Autodesk Inventor part; units mm, degrees
ref_plane "YZ Plane" through (0, 0, 0) normal (1, 0, 0) x (0, 1, 0)
ref_plane "XZ Plane" through (0, 0, 0) normal (0, 1, 0) x (-1, 0, 0)
ref_plane "XY Plane" through (0, 0, 0) normal (0, 0, 1) x (1, 0, 0)
sketch "Skizze2" plane through (0, 0, 0) normal (0, 0, 1) x (1, 0, 0)
  line L0 (-122.5, 30) -> (122.5, 30)
  line L1 (122.5, 30) -> (122.5, -30)
  line L2 (122.5, -30) -> (-122.5, -30)
  line L3 (-122.5, -30) -> (-122.5, 30)
  line L4 (-122.5, 30) -> (122.5, -30) construction
  line L5 (122.5, 30) -> (-122.5, -30) construction
  point P0 (0, 0)
  dimension "d0" = 245
  dimension "d1" = 60
extrude "Extrusion1" add sketch "Skizze2" along normal blind 2.5
sketch "Skizze3" plane through (0, 0, 2.5) normal (0, 0, 1) x (1, 0, 0)
  line L0 (122.5, 30) -> (-122.5, 30) construction
  line L1 (-122.5, 30) -> (-122.5, -30) construction
  line L2 (-122.5, -30) -> (122.5, -30) construction
  line L3 (122.5, -30) -> (122.5, 30) construction
  line L4 (122.5, 30) -> (-122.5, 30)
  line L5 (122.5, -30) -> (122.5, 30)
  line L6 (-122.5, 30) -> (122.5, 30)
  line L7 (122.5, 30) -> (122.5, 27.5)
  line L8 (122.5, 27.5) -> (-122.5, 27.5)
  line L9 (-122.5, 27.5) -> (-122.5, 30)
  point P0 (0, 0)
  dimension "d4" = 2.5
extrude "Extrusion2" add sketch "Skizze3" along normal blind 20
sketch "Skizze4" plane through (-122.5, 30, 0) normal (0, 1, 0) x (1, 0, 0)
  line L0 (0, 0) -> (245, 0) construction
  line L1 (0, 0) -> (0, -22.5) construction
  line L2 (245, -22.5) -> (0, -22.5) construction
  line L3 (245, 0) -> (245, -22.5) construction
  line L4 (122.5, 0) -> (7, 0) construction
  line L5 (0, 0) -> (245, 0) construction
  line L6 (7, 0) -> (238, 0) construction
  line L7 (7, -22.5) -> (7, -14.5) construction
  line L8 (245, -22.5) -> (0, -22.5)
  line L9 (238, -22.5) -> (238, -14.5) construction
  line L10 (7, -19.5) -> (7, -9.5) construction
  line L11 (9, -19.5) -> (9, -9.5)
  line L12 (5, -9.5) -> (5, -19.5)
  arc A0 (5, -19.5) -> (9, -19.5) centre (7, -19.5) ccw
  arc A1 (9, -9.5) -> (5, -9.5) centre (7, -9.5) ccw
  line L13 (238, -9.5) -> (238, -19.5) construction
  line L14 (236, -9.5) -> (236, -19.5)
  line L15 (240, -19.5) -> (240, -9.5)
  arc A2 (240, -9.5) -> (236, -9.5) centre (238, -9.5) ccw
  arc A3 (236, -19.5) -> (240, -19.5) centre (238, -19.5) ccw
  dimension "d8" = 231
  dimension "d9" = 8
  dimension "d10" = 5
  dimension "d11" = 4
  dimension "d12" = 8
  dimension "d13" = 5
  dimension "d14" = 4
extrude "Extrusion3" cut sketch "Skizze4" against normal blind 20
sketch "Skizze5" plane through (0, 0, 2.5) normal (0, 0, 1) x (1, 0, 0)
  line L0 (122.5, 27.5) -> (-122.5, 27.5) construction
  line L1 (-122.5, 27.5) -> (-122.5, -30) construction
  line L2 (-122.5, -30) -> (122.5, -30) construction
  line L3 (122.5, -30) -> (122.5, 27.5) construction
  line L4 (122.5, -30) -> (122.5, 27.5)
  line L5 (122.5, 27.5) -> (122.5, -30)
  line L6 (122.5, -30) -> (-122.5, -30)
  line L7 (-122.5, -30) -> (-122.5, 27.5)
  line L8 (-122.5, 24.8143) -> (-120.5, 24.8143) construction
  line L9 (122.5, 16.3856) -> (120.5, 16.3856) construction
  line L10 (-122.5, -30) -> (122.5, -30)
  line L11 (0, -30) -> (0, -28) construction
  line L12 (120.5, 27.5) -> (120.5, -28)
  line L13 (120.5, -28) -> (-120.5, -28)
  line L14 (-120.5, -28) -> (-120.5, 27.5)
  line L15 (-122.5, 27.5) -> (-120.5, 27.5)
  line L16 (120.5, 27.5) -> (122.5, 27.5)
  point P0 (0, 0)
  dimension "d17" = 2
  dimension "d18" = 2
  dimension "d19" = 2
extrude "Extrusion4" add sketch "Skizze5" along normal blind 8
fillet "Rundung1" radius 2 7 edges at (-122.5, 30, 11.25) (0, 30, 0) (122.5, 30, 11.25) (0, 30, 22.5) (122.5, 0, 0) (-122.5, 0, 0) (0, -30, 0)
sketch "Skizze7" plane through (0, 0, 0) normal (0, 0, -1) x (-1, 0, 0)
  line L0 (120.5, 30) -> (-120.5, 30) construction
  line L1 (122.5, -30) -> (122.5, 28) construction
  line L2 (-122.5, -30) -> (122.5, -30) construction
  line L3 (-122.5, 28) -> (-122.5, -30) construction
  line L4 (0, 30) -> (0, 0) construction
  line L5 (-102.5, 0.65) -> (102.5, 0.65)
  line L6 (102.5, 0.65) -> (102.5, -0.65)
  line L7 (102.5, -0.65) -> (-102.5, -0.65)
  line L8 (-102.5, -0.65) -> (-102.5, 0.65)
  line L9 (-102.5, 0.65) -> (102.5, -0.65) construction
  line L10 (102.5, 0.65) -> (-102.5, -0.65) construction
  dimension "d28" = 205
  dimension "d29" = 1.3
extrude "Extrusion6" cut sketch "Skizze7" against normal blind 5
sketch "Skizze8" plane through (0, 0, 2.5) normal (0, 0, 1) x (1, 0, 0)
  line L0 (102.5, -0.65) -> (-102.5, -0.65) construction
  line L1 (-102.5, -0.65) -> (102.5, -0.65)
  line L2 (102.5, -0.65) -> (102.5, -2.6532)
  line L3 (102.5, -2.6532) -> (-102.5, -2.6532)
  line L4 (-102.5, -2.6532) -> (-102.5, -0.65)
  point P0 (0, 0)
extrude "Extrusion7" add sketch "Skizze8" along normal blind 5
fillet "Rundung2" radius 2 2 edges at (-102.5, -1.6516, 7.5) (102.5, -1.6516, 7.5)
sketch "Skizze9" plane through (0, 0, 2.5) normal (0, 0, 1) x (1, 0, 0)
  line L0 (-102.5, 0.65) -> (102.5, 0.65) construction
  line L1 (100.5, -0.65) -> (-100.5, -0.65) construction
  line L2 (-102.5, 0.65) -> (102.5, 0.65)
  line L3 (102.5, 0.65) -> (102.5, 1.65)
  line L4 (102.5, 1.65) -> (-102.5, 1.65)
  line L5 (-102.5, 1.65) -> (-102.5, 0.65)
  point P0 (0, 0)
  dimension "d35" = 1
extrude "Extrusion8" cut sketch "Skizze9" against normal blind 10
sketch "Skizze10" plane through (0, 0, 2.5) normal (0, 0, 1) x (1, 0, 0)
  line L0 (-102.5, 1.65) -> (102.5, 1.65)
  line L1 (-102.5, 1.65) -> (102.5, 1.65)
  line L2 (102.5, 1.65) -> (102.5, 3.65)
  line L3 (102.5, 3.65) -> (-102.5, 3.65)
  line L4 (-102.5, 3.65) -> (-102.5, 1.65)
  point P0 (0, 0)
  dimension "d38" = 2
extrude "Extrusion9" add sketch "Skizze10" along normal blind 5
properties part number "Basket" material "Acetalharz, Schwarz"
Geometry: final body of the model. Coordinates: model frame, mm. A direction names the side the tool comes from. Coordinates: 2 decimals unless noted, no trailing zeros. Loops run counter-clockwise (first coordinate to the right, second up) from the corner with the lowest first, then second, coordinate; pieces in that order, holes last. Notation, with made-up numbers: (75, 7) -> (92, 7) arc R20 ccw to (92, 30) -> close; hole circle Ø8 at (-14, -2). An arc over 180 degrees is marked (long way). Use a Markdown table: item, result. Add a question column.
(1) Section query C-C, the plane y = 22. Return loops of the section in (x, z), plus the area to 3 significant figures.
(2) Access query for faces 1 (the flat face through (-1, -0.65, 4)), 2 (the flat face through (2, -28, 6)), 3 (the flat face through (2, -30, 6)). Directions: +Z, -Z, +X, -X, +Y, -Y. A direction counts if a zero-diameter tool reaches every point of the face in a straight line with its end or side. Return the directions, or none.
(3) Section query B-B, the plane x = -22.5. Return loops of the section in (y, z), plus the area to 3 significant figures.
(4) Pin query (flat end, axial travel): pin 1 Ø0.7 at (y, z) = (1, 1) entering from +X; pin 2 Ø1.2 at (y, z) = (29.5, 16) entering from +X; pin 3 Ø2 at (x, y) = (40, 3) entering from +Z. Return the tip coordinate at first contact, or that it passes through.
(5) Line query: line 1 along Y through (x, z) = (37.5, 5.75); line 2 along X through (y, z) = (16.5, 8.25); line 3 along Y through (x, z) = (-43, 8). Output: solid intervals per line, ascending.
(6) Section query A-A, the plane z = 13.5. Return loops of the section in (x, y).
(7) Mould query, pull axis X, two halves, no side actions, for faces 4 (the flat face through (-1, 1.65, 4)), 5 (the flat face through (-1, -29, 10.5)), 6 (the flat face through (122.5, -1, 5)). Classes: pulls with the +X half, pulls with the -X half, needs draft (parallel to the pull), parting line crosses it, or undercut.
Answer:
| question | item | result |
|---|---|---|
| 1 | outline | (-122.5, 2) arc R2 ccw to (-120.5, 0) -> (120.5, 0) arc R2 ccw to (122.5, 2) -> (122.5, 10.5) -> (120.5, 10.5) -> (120.5, 2.5) -> (-120.5, 2.5) -> (-120.5, 10.5) -> (-122.5, 10.5) -> close |
| 1 | area | 643 mm^2 |
| 2 | face 1 | +Z, -Z |
| 2 | face 2 | +Z |
| 2 | face 3 | +Z, -Z, +X, -X, -Y |
| 3 | outline | (-30, 2) arc R2 ccw to (-28, 0) -> (-0.65, 0) -> (-0.65, 7.5) -> (-2.65, 7.5) -> (-2.65, 2.5) -> (-28, 2.5) -> (-28, 10.5) -> (-30, 10.5) -> close; (1.65, 0) -> (28, 0) arc R2 ccw to (30, 2) -> (30, 20.5) arc R2 ccw to (28, 22.5) -> (27.5, 22.5) -> (27.5, 2.5) -> (3.65, 2.5) -> (3.65, 7.5) -> (1.65, 7.5) -> close |
| 3 | area | 228 mm^2 |
| 4 | pin 1 | stops at x = 122.39 |
| 4 | pin 2 | stops at x = 122.29 |
| 4 | pin 3 | stops at z = 7.5 |
| 5 | line 1 | y = -30 to -28, -2.65 to -0.65, 1.65 to 3.65, 27.5 to 30 |
| 5 | line 2 | x = -122.5 to -120.5, 120.5 to 122.5 |
| 5 | line 3 | y = -30 to -28, 27.5 to 30 |
| 6 | outline | (-122.5, 27.5) -> (-117.5, 27.5) -> (-117.5, 30) -> (-120.5, 30) arc R2 ccw to (-122.5, 28) -> close; (-113.5, 27.5) -> (113.5, 27.5) -> (113.5, 30) -> (-113.5, 30) -> close; (117.5, 27.5) -> (122.5, 27.5) -> (122.5, 28) arc R2 ccw to (120.5, 30) -> (117.5, 30) -> close |
| 7 | face 4 | undercut |
| 7 | face 5 | needs draft |
| 7 | face 6 | pulls with the +X half |
